Input: part model. Units: mm. Frame: model coordinates. Coordinates: 2 decimals unless noted, no trailing zeros. Loops run counter-clockwise (first coordinate to the right, second up) from the corner with the lowest first, then second, coordinate; pieces in that order, holes last.
Item 1: Pull-direction query (Z, two-part tool) for faces 1 (the flat face through (-0.1, 0.5, 8.7)), 2 (the flat face through (-0.3, 0.5, 12.5)), 3 (the cylindrical face through (-15.676, 0.507, -11.339)), 4 (the flat face through (0, 1, 10)); classes: released by +Z, released by -Z, zero draft, split by the parting line, or undercut.
Item 2: Section C-C on x = -2. Return loops of the section in (y, z).
Item 3: Section D-D on z = -10. Return loops of the section in (x, y).
Item 4: Ray query, line 1 along X through (y, z) = (0.65, -10); line 2 along Z through (x, y) = (-15.5, 0.3); line 3 along X through (y, z) = (0.1, -6). Return the intervals inside material, ascending.
Item 5: Contact query for flat-ended pins moving along their axis: P1, Ø9, axis at x = 1, z = -1.5, coming from the +Y side; P2, Ø8, axis at x = -1, z = 9, coming from the +Y side. Output: stop coordinate, or through.
Item 6: Section B-B on z = -6.5. Return loops of the section in (x, y).
Item 7: Section A-A on x = 15.5. Return loops of the section in (y, z).
```python
from build123d import *

# Parameters (mm, degrees)
SKETCH1_W           = 35.8
SKETCH1_H           = 25
SKETCH1_W_2         = 24
SKETCH1_H_2         = 16
BOSS_EXTRUDE1_DEPTH = 1
SKETCH2_W           = 26.2
SKETCH2_H           = 18.2
CUT_EXTRUDE1_DEPTH  = 0.5
CUT_EXTRUDE2_REACH  = 3
SKETCH3_R           = 1.35


with BuildPart() as part:
    # Sketch1 → Boss-Extrude1 (new body)
    with BuildSketch(Plane(origin=(0, 0, 0), x_dir=(1, 0, 0), z_dir=(0, 1, 0))):
        Rectangle(SKETCH1_W, SKETCH1_H)
        Rectangle(SKETCH1_W_2, SKETCH1_H_2, mode=Mode.SUBTRACT)
    extrude(amount=BOSS_EXTRUDE1_DEPTH)

    # Sketch2 → Cut-Extrude1 (cut)
    with BuildSketch(Plane(origin=(0, 1, 0), x_dir=(1, 0, 0), z_dir=(0, 1, 0))):
        Rectangle(SKETCH2_W, SKETCH2_H)
    extrude(amount=-CUT_EXTRUDE1_DEPTH, mode=Mode.SUBTRACT)

    # Sketch3 → Cut-Extrude2 (cut, up to next)
    with BuildSketch(Plane(origin=(0, 1, 0), x_dir=(1, 0, 0), z_dir=(0, 1, 0)), mode=Mode.PRIVATE) as cut_extrude2_sk1:
        with Locations((-15.5, 10)):
            Circle(SKETCH3_R)
    cut_extrude2_tool1 = extrude(cut_extrude2_sk1.sketch, amount=-CUT_EXTRUDE2_REACH, mode=Mode.PRIVATE) & part.part
    add(cut_extrude2_tool1.solids().sort_by_distance((-15.5, 1, -10))[0], mode=Mode.SUBTRACT)
    # Sketch3 → Cut-Extrude2 (cut, up to next)
    with BuildSketch(Plane(origin=(0, 1, 0), x_dir=(1, 0, 0), z_dir=(0, 1, 0)), mode=Mode.PRIVATE) as cut_extrude2_sk2:
        with Locations((-15.5, -10)):
            Circle(SKETCH3_R)
    cut_extrude2_tool2 = extrude(cut_extrude2_sk2.sketch, amount=-CUT_EXTRUDE2_REACH, mode=Mode.PRIVATE) & part.part
    add(cut_extrude2_tool2.solids().sort_by_distance((-15.5, 1, 10))[0], mode=Mode.SUBTRACT)
    # Sketch3 → Cut-Extrude2 (cut, up to next)
    with BuildSketch(Plane(origin=(0, 1, 0), x_dir=(1, 0, 0), z_dir=(0, 1, 0)), mode=Mode.PRIVATE) as cut_extrude2_sk3:
        with Locations((15.5, -10)):
            Circle(SKETCH3_R)
    cut_extrude2_tool3 = extrude(cut_extrude2_sk3.sketch, amount=-CUT_EXTRUDE2_REACH, mode=Mode.PRIVATE) & part.part
    add(cut_extrude2_tool3.solids().sort_by_distance((15.5, 1, 10))[0], mode=Mode.SUBTRACT)
    # Sketch3 → Cut-Extrude2 (cut, up to next)
    with BuildSketch(Plane(origin=(0, 1, 0), x_dir=(1, 0, 0), z_dir=(0, 1, 0)), mode=Mode.PRIVATE) as cut_extrude2_sk4:
        with Locations((15.5, 10)):
            Circle(SKETCH3_R)
    cut_extrude2_tool4 = extrude(cut_extrude2_sk4.sketch, amount=-CUT_EXTRUDE2_REACH, mode=Mode.PRIVATE) & part.part
    add(cut_extrude2_tool4.solids().sort_by_distance((15.5, 1, -10))[0], mode=Mode.SUBTRACT)


solid = part.part
```
Results found:
1. face 1: undercut
1. face 2: released by +Z
1. face 3: undercut
1. face 4: zero draft
2. outline: (0, -12.5) - (1, -12.5) - (1, -9.1) - (0.5, -9.1) - (0.5, -8) - (0, -8) - close; (0, 8) - (0.5, 8) - (0.5, 9.1) - (1, 9.1) - (1, 12.5) - (0, 12.5) - close
3. outline: (-17.9, 0) - (-16.85, 0) - (-16.85, 1) - (-17.9, 1) - close; (-14.15, 0) - (14.15, 0) - (14.15, 1) - (-14.15, 1) - close; (16.85, 0) - (17.9, 0) - (17.9, 1) - (16.85, 1) - close
4. line 1: x = -17.9 to -16.85, -14.15 to 14.15, 16.85 to 17.9
4. line 2: z = -12.5 to -11.35, -8.65 to 8.65, 11.35 to 12.5
4. line 3: x = -17.9 to -12, 12 to 17.9
5. P1: passes through
5. P2: stops at y = 1
6. outline: (-17.9, 0) - (-12, 0) - (-12, 0.5) - (-13.1, 0.5) - (-13.1, 1) - (-17.9, 1) - close; (12, 0) - (17.9, 0) - (17.9, 1) - (13.1, 1) - (13.1, 0.5) - (12, 0.5) - close
7. outline: (0, -12.5) - (1, -12.5) - (1, -11.35) - (0, -11.35) - close; (0, -8.65) - (1, -8.65) - (1, 8.65) - (0, 8.65) - close; (0, 11.35) - (1, 11.35) - (1, 12.5) - (0, 12.5) - close
